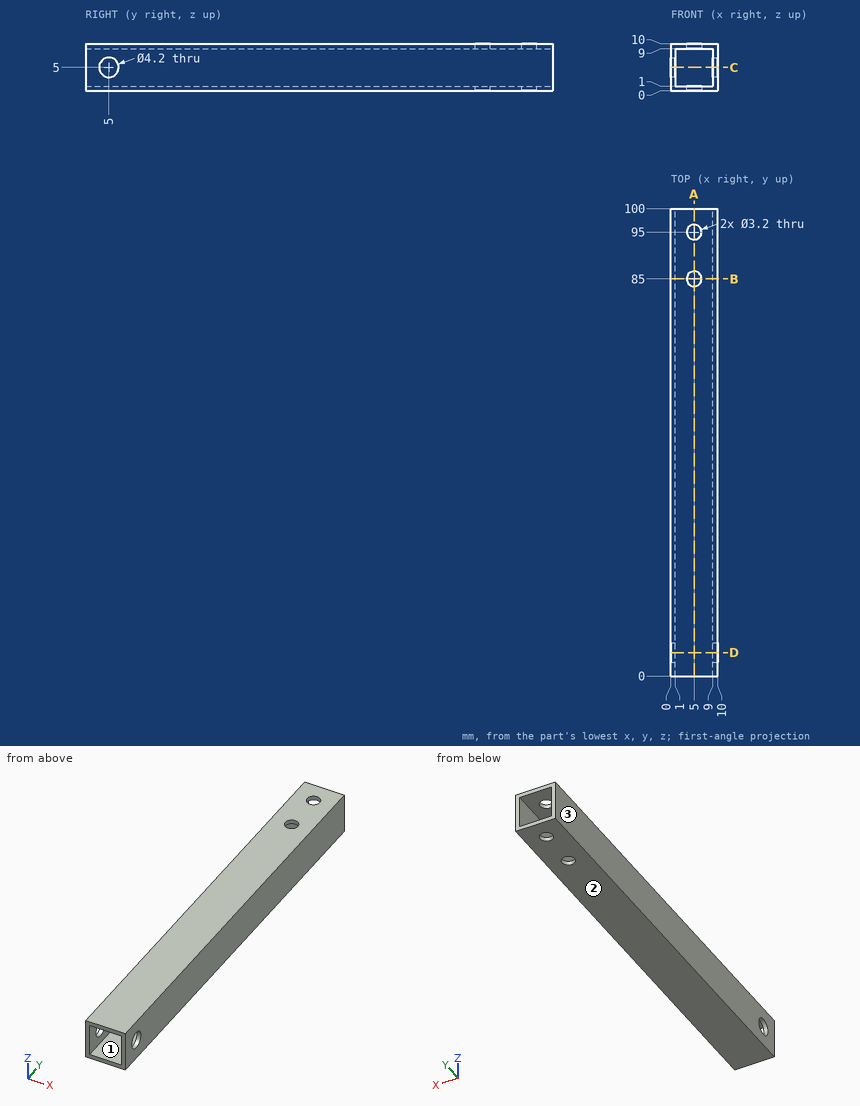
Geometry check sheet. Reference: drawing and pictorial views, mm from the part's lowest x, y, z. Give positions to 0.01 mm unless a question says otherwise; leave off trailing zeros. Order: outer loops, then holes, each group sorted by start corner. A loop starts at its lowest first (then second) coordinate and runs counter-clockwise, first axis right, second up.
1. Section check B-B, the plane y = 85. Enter the section's corners in (x, z).
2. Section check A-A, the plane x = 5. Enter the section's corners in (y, z), and give its area (3 significant figures).
3. Section check C-C, the plane z = 5. Enter the section's corners in (x, y), and give its area (3 significant figures).
4. Thickness scan on L1, parallel to Y at x = 5, z = 0.3; L2, parallel to Y at x = 0.55, z = 5; L3, parallel to Z at x = 2, y = 18. Record the ranges inside material, lowest first.
5. Section check D-D, the plane y = 5. Enter the section's corners in (x, z).
6. Release check for a two-part mould opening along Z. For the marked faces 1, 2 and 3 record: pulls with the +Z half, pulls with the -Z half, needs draft (parallel to the pull), parting line crosses it, or undercut.
Values follow:
1. outline: (0, 0) - (3.4, 0) - (3.4, 1) - (1, 1) - (1, 9) - (3.4, 9) - (3.4, 10) - (0, 10) - close; (6.6, 0) - (10, 0) - (10, 10) - (6.6, 10) - (6.6, 9) - (9, 9) - (9, 1) - (6.6, 1) - close
2. outline: (0, 0) - (83.4, 0) - (83.4, 1) - (0, 1) - close; (0, 9) - (83.4, 9) - (83.4, 10) - (0, 10) - close; (86.6, 0) - (93.4, 0) - (93.4, 1) - (86.6, 1) - close; (86.6, 9) - (93.4, 9) - (93.4, 10) - (86.6, 10) - close; (96.6, 0) - (100, 0) - (100, 1) - (96.6, 1) - close; (96.6, 9) - (100, 9) - (100, 10) - (96.6, 10) - close
2. area: 187 mm2
3. outline: (0, 0) - (1, 0) - (1, 2.9) - (0, 2.9) - close; (0, 7.1) - (1, 7.1) - (1, 100) - (0, 100) - close; (9, 0) - (10, 0) - (10, 2.9) - (9, 2.9) - close; (9, 7.1) - (10, 7.1) - (10, 100) - (9, 100) - close
3. area: 192 mm2
4. L1: y = 0 to 83.4, 86.6 to 93.4, 96.6 to 100
4. L2: y = 0 to 2.9, 7.1 to 100
4. L3: z = 0 to 1, 9 to 10
5. outline: (0, 0) - (10, 0) - (10, 2.9) - (9, 2.9) - (9, 1) - (1, 1) - (1, 2.9) - (0, 2.9) - close; (0, 7.1) - (1, 7.1) - (1, 9) - (9, 9) - (9, 7.1) - (10, 7.1) - (10, 10) - (0, 10) - close
6. face 1: undercut
6. face 2: pulls with the -Z half
6. face 3: needs draft
